from build123d import *

# Parameters (mm, degrees)
F1_DEPTH = 9.1
F3_DEPTH = 10


with BuildPart() as f1:
    # F0 (on Top) → F1 (new body)
    with BuildSketch(Plane.XY):
        with BuildLine():
            Line((-45.512, 26.294801), (-50.512, 26.294801))
            Line((-50.512, 26.294801), (-50.512, -33.705199))
            Line((-50.512, -33.705199), (-0.512, -33.705199))
            Line((-0.512, -33.705199), (-0.512, 26.294801))
            Line((-0.512, 26.294801), (-5.512, 26.294801))
            ThreePointArc((-5.512, 26.294801), (-25.512, 6.294801), (-45.512, 26.294801))
        make_face()
    extrude(amount=F1_DEPTH)

    # F2 (on face) → F3 (join)
    with BuildSketch(Plane.XZ.offset(33.705199)):
        Polygon((-0.512, 0), (-50.512, 0), (-35.512, -34.577517), (-15.512, -34.577517), align=None)
        with BuildLine():
            ThreePointArc((-28.124191, -7.687931), (-25.512, -5.075741), (-22.89981, -7.687931))
            Line((-22.89981, -7.687931), (-22.89981, -18.501936))
            ThreePointArc((-22.89981, -18.501936), (-25.512, -21.114126), (-28.124191, -18.501936))
            Line((-28.124191, -18.501936), (-28.124191, -7.687931))
        make_face(mode=Mode.SUBTRACT)
    extrude(amount=-F3_DEPTH)


solid = f1.part
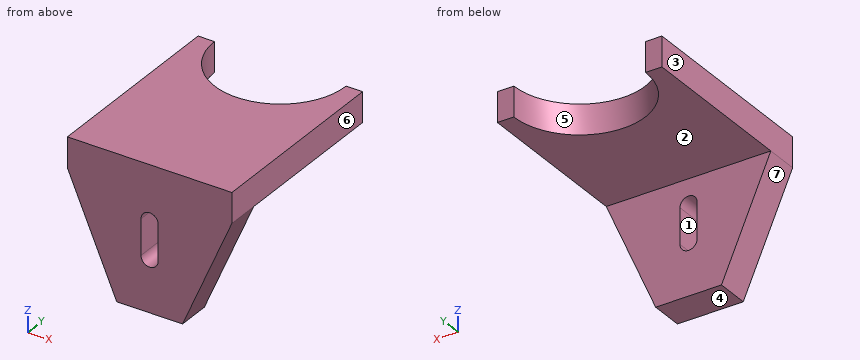
For this review, take the finished solid that the model builds, in its own axes (mm). Face numbers are marked on the shaded views. A direction names the side the tool comes from. Coordinates: 2 decimals unless noted, no trailing zeros. Order: outer loops, then holes, each group sorted by start corner. A loop starts at its lowest first (then second) coordinate and runs counter-clockwise, first axis right, second up. Notation, with made-up numbers: (77, 34) - (111, 34) arc R23 cw to (111, 51) - close; hole circle Ø5 at (-17.75, 22.5). An arc over 180 degrees is marked (long way). Answer as CSV lines item,"result". Start each with the question number.
1) Add section C-C (x = -26). State the section outline as (y, z) points.
2) To check wall thickness, follow line 1 along Z through (x, y) = (-42, 6); line 2 along X through (y, z) = (14, 4); line 3 along Y through (x, z) = (-29.5, -25). State the ranges of each line that lie inside material, in increasing order. Write a range as [from, to].
3) Add section B-B (z = -14). State the section outline as (x, y) points, then the cut area to 3 significant figures.
4) Add section D-D (z = 2.5). State the section outline as (x, y) points, then the cut area to 3 significant figures.
5) Insertion check: P1, Ø5, axis at y = -30.5, z = -11, coming from the +X side; P2, Ø12, axis at x = -29.5, z = -22, coming from the +Y side; P3, Ø12, axis at x = -37, z = 4, coming from the +Y side; P4, Ø10, axis at x = -42.5, z = -24, coming from the -Y side. Each pin has a flat end and moves straight along its axis. Give the tip position at first contact, or say it passes through.
6) Machinability: for the marked faces 1, 2 and 3, which of the approach directions +Z, -Z, +X, -X, +Y, -Y give a long, thin tool a straight path to every point of the face, cutting with its end or side? Answer none if there is none.
7) Draft analysis for pull direction X (two halves, no side actions). For the marked faces 4, 5, 6 and 7, state which applies: +X half, -X half, draft (parallel to the pull), parting line (faces both ways), or undercut.
8) Add section A-A (y = 23). State the section outline as (x, z) points.
Result:
1,outline,"(-33.71, -34.58) - (-23.71, -34.58) - (-23.71, -21.07) - (-33.71, -21.07) - close; (-33.71, -5.12) - (-23.71, -5.12) - (-23.71, 0) - (6.3, 0) - (6.3, 9.1) - (-33.71, 9.1) - close"
2,line 1,"[0, 9.1]"
2,line 2,"[-50.51, -41.29], [-9.74, -0.51]"
2,line 3,"[-33.71, -23.71]"
3,outline,"(-44.44, -33.71) - (-28.12, -33.71) - (-28.12, -23.71) - (-44.44, -23.71) - close; (-22.9, -33.71) - (-6.59, -33.71) - (-6.59, -23.71) - (-22.9, -23.71) - close"
3,area,"326 mm^2"
4,outline,"(-50.51, -33.71) - (-0.51, -33.71) - (-0.51, 26.29) - (-5.51, 26.29) arc R20 cw to (-45.51, 26.29) - (-50.51, 26.29) - close"
4,area,"2,370 mm^2"
5,P1,"x = -4.2"
5,P2,"y = -23.71"
5,P3,"y = 16.59"
5,P4,"y = -33.71"
6,face 1,"+Y, -Y"
6,face 2,"-Z, +X, -X, +Y"
6,face 3,"+Z, -Z, -X, +Y, -Y"
7,face 4,"draft"
7,face 5,"undercut"
7,face 6,"+X half"
7,face 7,"-X half"
8,outline,"(-50.51, 0) - (-45.24, 0) - (-45.24, 9.1) - (-50.51, 9.1) - close; (-5.79, 0) - (-0.51, 0) - (-0.51, 9.1) - (-5.79, 9.1) - close"
